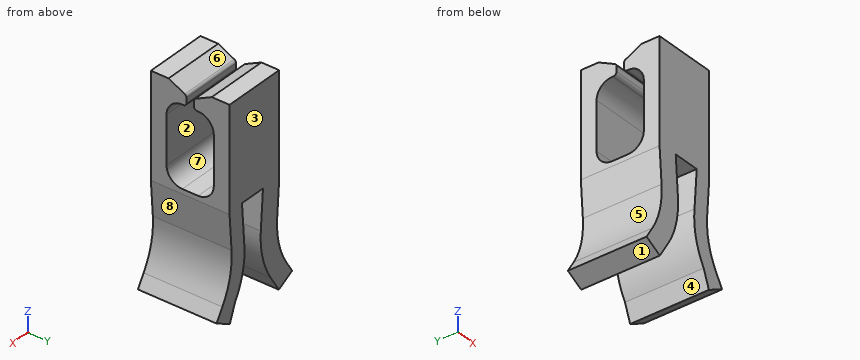
from build123d import *

# Parameters (mm, degrees)
F1_DEPTH = 5
F3_DEPTH = 5.048269


with BuildPart() as f1:
    # F0 (on Front) → F1 (new body)
    with BuildSketch(Plane.XZ):
        with BuildLine():
            Line((0, 13.115867), (-2, 13.115867))
            Line((-2, 13.115867), (-2, 6.558903))
            Line((-2, 6.558903), (-1.838625, 4.335265))
            ThreePointArc((-1.838625, 4.335265), (-1.97121, 2.77512), (-2.579833, 1.33248))
            Line((-2.579833, 1.33248), (-3.047269, 0.580993))
            Line((-3.047269, 0.580993), (-1.976246, 0))
            Line((-1.976246, 0), (-1.304174, 1.080476))
            ThreePointArc((-1.304174, 1.080476), (-0.659034, 2.609675), (-0.518494, 4.263429))
            Line((-0.518494, 4.263429), (-0.696581, 6.717356))
            Line((-0.696581, 6.717356), (0, 6.717356))
            Line((0, 6.717356), (0, 13.115867))
        make_face()
        with BuildLine():
            Line((2, 13.115867), (0, 13.115867))
            Line((0, 13.115867), (0, 6.717356))
            Line((0, 6.717356), (0.99737, 6.717356))
            Line((0.99737, 6.717356), (0.817707, 4.241714))
            ThreePointArc((0.817707, 4.241714), (0.924554, 2.599253), (1.558914, 1.080476))
            Line((1.558914, 1.080476), (1.976246, 0))
            Line((1.976246, 0), (3.047269, 0.580993))
            Line((3.047269, 0.580993), (2.579833, 1.33248))
            ThreePointArc((2.579833, 1.33248), (1.97121, 2.77512), (1.838625, 4.335265))
            Line((1.838625, 4.335265), (2, 6.558903))
            Line((2, 6.558903), (2, 13.115867))
        make_face()
    extrude(amount=F1_DEPTH)

    # F2 (on face) → F3 (cut, through all)
    with BuildSketch(Plane.YZ.offset(2)):
        with BuildLine():
            ThreePointArc((-2.844955, 12.600366), (-2.764493, 12.526635), (-2.734718, 12.421641))
            Line((-2.734718, 12.421641), (-2.734718, 12.105381))
            ThreePointArc((-2.734718, 12.105381), (-2.793296, 11.963959), (-2.934718, 11.905381))
            Line((-2.934718, 11.905381), (-3, 11.905381))
            ThreePointArc((-3, 11.905381), (-3.707107, 11.612487), (-4, 10.905381))
            Line((-4, 10.905381), (-4, 7.860531))
            ThreePointArc((-4, 7.860531), (-3.707107, 7.153424), (-3, 6.860531))
            Line((-3, 6.860531), (-2.5, 6.860531))
            Line((-2.5, 6.860531), (-2, 6.860531))
            ThreePointArc((-2, 6.860531), (-1.292893, 7.153424), (-1, 7.860531))
            Line((-1, 7.860531), (-1, 10.905381))
            ThreePointArc((-1, 10.905381), (-1.292893, 11.612487), (-2, 11.905381))
            Line((-2, 11.905381), (-2.065282, 11.905381))
            ThreePointArc((-2.065282, 11.905381), (-2.206704, 11.963959), (-2.265282, 12.105381))
            Line((-2.265282, 12.105381), (-2.265282, 12.421641))
            ThreePointArc((-2.265282, 12.421641), (-2.235507, 12.526635), (-2.155045, 12.600366))
            Line((-2.155045, 12.600366), (-1.128649, 13.115867))
            Line((-1.128649, 13.115867), (-2.5, 13.115867))
            Line((-2.5, 13.115867), (-3.871351, 13.115867))
            Line((-3.871351, 13.115867), (-2.844955, 12.600366))
        make_face()
    extrude(amount=-F3_DEPTH, mode=Mode.SUBTRACT)


solid = f1.part
For this review, take the finished solid that the model builds, in its own axes (mm). Face numbers are marked on the shaded views. A direction names the side the tool comes from. Round coordinates to 2 decimals unless told otherwise and drop trailing zeros. Order: outer loops, then holes, each group sorted by start corner. A loop starts at its lowest first (then second) coordinate and runs counter-clockwise, first axis right, second up. Notation, with made-up numbers: M 32.25,-11.5 L 68.25,-11.5 A9 cw 68.25,4.5 Z; hole C -6.75,-3.75 d10. An arc over 180 degrees is marked long. Use a Markdown table: item, result. Add a question column.
Item 1: Mouldability with a two-part tool opening along Y and no side actions: class the marked faces 1, 2 and 3 as released by +Y, released by -Y, zero draft, split by the parting line, or undercut.
Item 2: Add section C-C, the plane y = -1.8. Give the boundary of the cut face in (x, z).
Item 3: Tool access review of the marked faces 4, 5, 6, 7 and 8: name each direction out of +Z, -Z, +X, -X, +Y, -Y from which nothing blocks a thin tool from reaching the whole face with its end or side.
Item 4: Add section A-A, the plane z = 12.25. Give the boundary of the cut face in (x, y), then the cut area to 3 significant figures.
Item 5: To check wall thickness, follow line 1 along Y through (x, z) = (0.5, 9.75); line 2 along X through (y, z) = (-4.55, 3); line 3 along X through (y, z) = (-1, 11.5). State the ranges of each line that lie inside material, in increasing order.
Item 6: Add section B-B, the plane y = -4.4. Give the boundary of the cut face in (x, z).
Item 7: Insertion check: pin 1 (2.5 mm diameter, centred on y = -3, z = 11, fed in from -X); pin 2 (1.9 mm diameter, centred on x = 0, y = -3, fed in from -Z); pin 3 (3 mm diameter, centred on x = 0, y = -4, fed in from -Z). Each pin has a flat end and moves straight along its axis. Give the tip position at first contact, or say it passes through.
Item 8: Add section D-D, the plane z = 5.25. Give the boundary of the cut face in (x, y) (3 decimals), then the cut area to 3 significant figures.
Geometry results:
| question | item | result |
|---|---|---|
| 1 | face 1 | zero draft |
| 1 | face 2 | undercut |
| 1 | face 3 | released by +Y |
| 2 | outline | M -3.05,0.58 L -1.98,0 L -1.3,1.08 A5.3 ccw -0.52,4.26 L -0.7,6.72 L 1,6.72 L 0.82,4.24 A5 ccw 1.56,1.08 L 1.98,0 L 3.05,0.58 L 2.58,1.33 A5 cw 1.84,4.34 L 2,6.56 L 2,6.88 L -2,6.88 L -2,6.56 L -1.84,4.34 A5 cw -2.58,1.33 Z; M -2,11.89 L 2,11.89 L 2,12.78 L -2,12.78 Z |
| 3 | face 4 | -Z, +Y, -Y |
| 3 | face 5 | -X, +Y, -Y |
| 3 | face 6 | +Z, +X, -X |
| 3 | face 7 | +X, -X |
| 3 | face 8 | +X, +Y, -Y |
| 4 | outline | M -2,-5 L 2,-5 L 2,-2.73 L -2,-2.73 Z; M -2,-2.27 L 2,-2.27 L 2,0 L -2,0 Z |
| 4 | area | 18.1 mm² |
| 5 | line 1 | y = -5 to -4, -1 to 0 |
| 5 | line 2 | x = -1.92 to -0.58, 0.85 to 1.92 |
| 5 | line 3 | x = -2 to 2 |
| 6 | outline | M -3.05,0.58 L -1.98,0 L -1.3,1.08 A5.3 ccw -0.52,4.26 L -0.7,6.72 L 1,6.72 L 0.82,4.24 A5 ccw 1.56,1.08 L 1.98,0 L 3.05,0.58 L 2.58,1.33 A5 cw 1.84,4.34 L 2,6.56 L 2,13.12 L -2,13.12 L -2,6.56 L -1.84,4.34 A5 cw -2.58,1.33 Z |
| 7 | pin 1 | stops at x = -2 |
| 7 | pin 2 | stops at z = 1.75 |
| 7 | pin 3 | stops at z = 0.77 |
| 8 | outline | M -1.905,-5 L -0.59,-5 L -0.59,0 L -1.905,0 Z; M 0.891,-5 L 1.905,-5 L 1.905,0 L 0.891,0 Z |
| 8 | area | 11.6 mm² |
